Can you work these out from the drawing? Everything is in mm from the part's minimum corner. A direction names the side the tool comes from. Give positions to 0.01 mm unless a question says otherwise; leave off trailing zeros. Loops run counter-clockwise (first coordinate to the right, second up) from the corner with the lowest first, then second, coordinate; pieces in that order, holes last. Notation, with made-up numbers: (62, -18) - (76, -18) arc R37 cw to (76, 20) - close; hole circle Ø3 at (32.5, 15.25). An arc over 180 degrees is marked (long way). One line per item, written item: value. Start each with the question number.
Q1. I want a section at D-D (y = 26.5). Please give me the cut outline in (x, z).
Q2. If I drill on line 1 (X direction, y = 5, z = 25); line 2 (X direction, y = 17, z = 14); line 3 (Y direction, x = 8.5, z = 15.5), over which ranges is the centre line in solid material (lowest first)? Write a range as from..to.
Q3. I want a section at C-C (x = 32.5). Please give me the cut outline in (y, z) (3 decimals).
Q4. For the marked faces 1 and 2, which set-ups out of +Z, -Z, +X, -X, +Y, -Y let a thin tool reach every point of the face, with its end or its side?
Q5. I want a section at B-B (z = 4). Please give me the cut outline in (x, y), then the cut area to 3 significant figures.
Q6. I'm going to push flat-ended pins straight in: P1, Ø2, axis at y = 26.5, z = 3, coming from the +X side; P2, Ø10, axis at x = 26, z = 4.5, coming from the +Y side; P3, Ø1.5, axis at x = 43.5, z = 11, coming from the -Y side. Where does each tip first touch, or does it pass through?
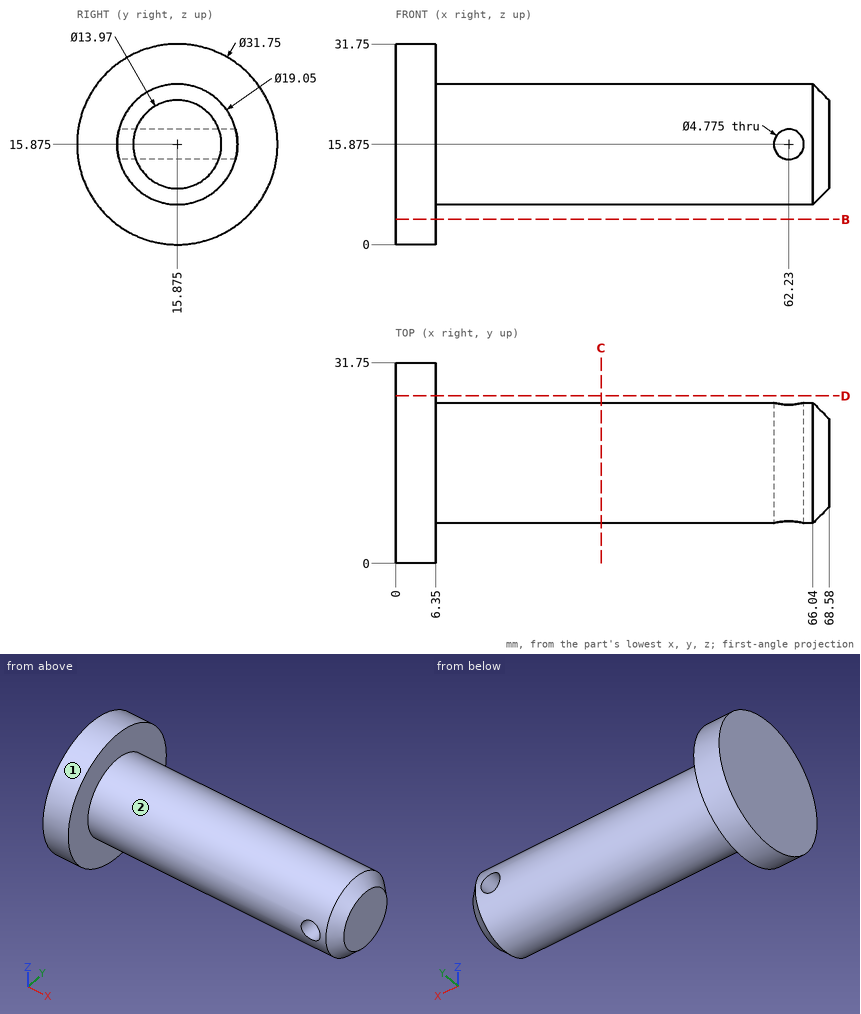
Worked answers:
1. outline: (0, 4.08) - (6.35, 4.08) - (6.35, 27.67) - (0, 27.67) - close
2. line 1: x = 0..6.35
2. line 2: x = 0..60.75, 63.71..68.58
2. line 3: y = 6.36..25.39
3. outline: circle Ø19.05 at (15.875, 15.875)
4. face 1: +X, -X
4. face 2: +X
5. outline: (0, 5.34) - (6.35, 5.34) - (6.35, 26.41) - (0, 26.41) - close
5. area: 134 mm²
6. P1: stops at x = 6.35
6. P2: stops at y = 22.95
6. P3: stops at y = 7.29
